Autodesk Inventor part; units mm, degrees
ref_plane "YZ Plane" through (0, 0, 0) normal (1, 0, 0) x (0, 1, 0)
ref_plane "XZ Plane" through (0, 0, 0) normal (0, 1, 0) x (-1, 0, 0)
ref_plane "XY Plane" through (0, 0, 0) normal (0, 0, 1) x (1, 0, 0)
sketch "Sketch1" plane through (0, 0, 0) normal (0, 1, 0) x (-1, 0, 0)
  circle A0 centre (0, 0) radius 39.95
  circle A1 centre (0, 0) radius 35.05
  line L0 (0, 0) -> (0, -5.05)
  line L1 (0, -5.05) -> (60, -5.05)
  line L2 (60, -5.05) -> (60, 5.05)
  line L3 (60, 5.05) -> (0, 5.05)
  line L4 (0, 5.05) -> (0, -5.05)
  line L5 (0, -5.05) -> (60, -5.05)
  line L6 (60, -5.05) -> (60, -8.05)
  line L7 (60, -8.05) -> (0, -8.05)
  line L8 (0, -8.05) -> (0, -5.05)
  line L9 (0, 5.05) -> (60, 5.05)
  line L10 (60, 5.05) -> (60, 8.05)
  line L11 (60, 8.05) -> (0, 8.05)
  line L12 (0, 8.05) -> (0, 5.05)
  line L13 (39.95, 0) -> (44.95, 0)
  line L14 (44.95, 0) -> (44.95, -8.05)
  line L15 (44.95, 0) -> (44.95, 8.05)
  point P0 (34.113, 8.05)
  point P1 (34.113, -8.05)
  point P2 (44.95, -5.05)
  point P3 (34.6843, -5.05)
  point P4 (34.6843, 5.05)
  point P5 (44.95, 5.05)
  point P6 (39.6295, 5.05)
  point P7 (39.6295, -5.05)
  dimension "d0" = 79.9
  dimension "d1" = 70.1
  dimension "d2" = 5.05
  dimension "d3" = 60
  dimension "d4" = 10.1
  dimension "d5" = 60
  dimension "d6" = 3
  dimension "d7" = 60
  dimension "d8" = 3
  dimension "d9" = 5
extrude "Extrusion1" add sketch "Sketch1" along normal blind 4.2 contours A0 L1 A1 L3 | L13 L14 L1 A0 | A0 L3 L15 L13 | L3 A1 L11 A0 | A0 L11 L15 L3 | L1 L14 L7 A0 | A0 L7 A1 L1
extrude "Extrusion2" add sketch "Sketch1" against normal blind 2 contours L3 A1 L11 A0 | A0 L11 L15 L3 | L1 L14 L7 A0 | A0 L7 A1 L1
extrude "Extrusion3" cut sketch "Sketch1" along normal blind 1 contours L13 L14 L1 A0 | A0 L3 L15 L13
sketch "Sketch4" plane through (-44.95, 4.2, 8.05) normal (0, 0, 1) x (1, 0, 0)
  line L0 (0, 0) -> (10.837, 0)
  line L1 (10.837, 0) -> (0, 0)
  line L2 (0, 0) -> (0, 2.5)
  line L3 (0, 2.5) -> (10.837, 2.5)
  line L4 (10.837, 2.5) -> (10.837, 0)
  line L5 (0, 2.5) -> (-30, 2.5)
  line L6 (-30, 2.5) -> (-30, 0)
  line L7 (-30, 0) -> (0, 0)
  line L8 (0, 0) -> (0, 2.5)
  line L9 (-30, 2.5) -> (-32.5, 2.5)
  line L10 (-32.5, 2.5) -> (-32.5, -6.2)
  line L11 (-32.5, -6.2) -> (-30, -6.2)
  line L12 (-30, -6.2) -> (-30, 2.5)
  line L13 (-32.5, -6.2) -> (-44.75, -6.2)
  line L14 (-44.75, -6.2) -> (-44.75, -3.7)
  line L15 (-44.75, -3.7) -> (-32.5, -3.7)
  line L16 (-32.5, -3.7) -> (-32.5, -6.2)
  point P0 (44.95, -4.2)
  point P1 (-30, 0)
  point P2 (-32.5, -3.7)
  dimension "d26" = 2.5
  dimension "d27" = 30
  dimension "d28" = 2.5
  dimension "d29" = 8.7
  dimension "d30" = 2.5
  dimension "d31" = 12.25
extrude "Extrusion6" add sketch "Sketch4" against normal up to surface (16.1 mm away)
sketch "Sketch5" plane through (-74.95, 4.2, 8.05) normal (0, -1, 0) x (1, 0, 0)
  line L0 (30, -16.1) -> (30, 0)
  line L1 (30, -8.05) -> (-8.75, -8.05)
  circle A0 centre (-8.75, -8.05) radius 3
  point P0 (74.95, -8.05)
  dimension "d34" = 38.75
  dimension "d35" = 6
extrude "Extrusion7" cut sketch "Sketch5" along normal blind 10
fillet "Fillet1" radius 5.5 2 edges at (-77.45, 6.7, 0) (-74.95, -2, 0)
fillet "Fillet2" radius 3 2 edges at (-74.95, 4.2, 0) (-77.45, 0.5, 0)
properties part number "measuring_support1"
Check sheet for the modelled part. Datum: model origin and axes. Units: mm. A direction names the side the tool comes from. Coordinates: 2 decimals unless noted, no trailing zeros. Write each loop counter-clockwise with the first axis right and the second up, starting at its lowest first coordinate (ties: lowest second). Pieces come first, ordered by that corner, then holes. Notation, with made-up numbers: (-30.75, -19.75) -> (20.25, -19.75) arc R33 ccw to (20.25, 15.25) -> close; hole circle Ø2 at (-15.75, -35). An arc over 180 degrees is marked (long way). Use a Markdown table: item, result.
1. Sectioned sample at B-B (x = -59). Enter the section's corners in (y, z), plus the area to 4 significant figures.
Reported:
| item | result |
|---|---|
| outline | (4.2, -8.05) -> (6.7, -8.05) -> (6.7, 8.05) -> (4.2, 8.05) -> close |
| area | 40.25 mm2 |
2. Tool access check on faces 4 (the cylindrical face through (-77.089, -0.853, -0.113)), 5 (the cylindrical face through (-35.05, 1.75, 0.11)), 6 (the cylindrical face through (-39.95, 0.49, 0.07)). Record the directions out of +Z, -Z, +X, -X, +Y, -Y that give a thin tool (end or side, any length) a straight path to the whole face; none if there is none.
Reported:
| item | result |
|---|---|
| face 4 | +Z, -Z, -Y |
| face 5 | +X, -Y |
| face 6 | -Y |
3. Go/stop test with flat-tipped pins: pin 1 Ø3 at (y, z) = (1, 3) entering from +X; pin 2 Ø9.5 at (x, z) = (-83.7, 0) entering from +Y; pin 3 Ø0.7 at (x, z) = (-34.5, 0) entering from -Y; pin 4 Ø2 at (x, y) = (-52.5, 3.5) entering from +Z. Record where each tip stops, or that it passes through.
Reported:
| item | result |
|---|---|
| pin 1 | stops at x = -34.76 |
| pin 2 | stops at y = 0.74 |
| pin 3 | stops at y = 4.2 |
| pin 4 | stops at z = 8.05 |
4. Scan lines: line 1 along Z through (x, y) = (-83.7, -1.45); line 2 along Y through (x, z) = (-55, 2); line 3 along X through (y, z) = (-0.75, 0). Record each from-to range of solid material in increasing order.
Reported:
| item | result |
|---|---|
| line 1 | z = -8.05 to -3, 3 to 8.05 |
| line 2 | y = 4.2 to 6.7 |
| line 3 | x = -89.7 to -86.7, -80.7 to -76.96 |
5. Release check for a two-part mould opening along X. For faces 1 (the cylindrical face through (-75.311, 5.553, -0.113)), 2 (the flat face through (-42, 1, 0)), 3 (the flat face through (-39, -2, 7)) record: pulls with the +X half, pulls with the -X half, needs draft (parallel to the pull), parting line crosses it, or undercut.
Reported:
| item | result |
|---|---|
| face 1 | pulls with the -X half |
| face 2 | undercut |
| face 3 | needs draft |
6. Sectioned sample at A-A (x = -83.7). Enter the section's corners in (y, z).
Reported:
| item | result |
|---|---|
| outline | (-2, -8.05) -> (0.5, -8.05) -> (0.5, -3) -> (-2, -3) -> close; (-2, 3) -> (0.5, 3) -> (0.5, 8.05) -> (-2, 8.05) -> close |
